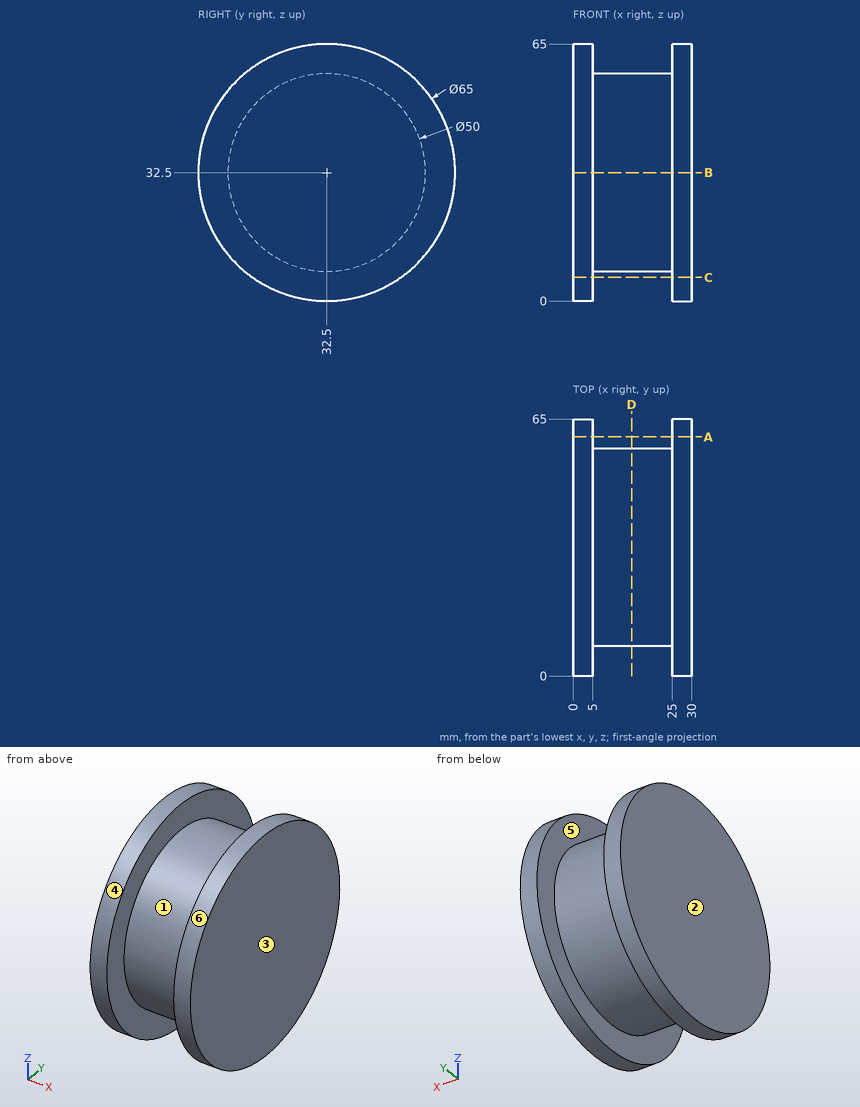
For this review, use the dimensioned drawing (mm, ordinates from the lowest corner) and the shaded views. A direction names the side the tool comes from. Round coordinates to 2 decimals unless told otherwise and drop trailing zeros. Loops run counter-clockwise (first coordinate to the right, second up) from the corner with the lowest first, then second, coordinate; pieces in that order, holes last. Notation, with made-up numbers: M -28.75,-13 L 17.25,-13 A24 cw 17.25,20 Z; hole C 88,8.5 d5. An arc over 180 degrees is marked long. Answer as a JSON object with one key per item and string values.
(1) Take a section at C-C on z = 6. Give the boundary of the cut face in (x, y).
Resolved:
{"outline": "M 0,13.69 L 5,13.69 L 5,51.31 L 0,51.31 Z; M 25,13.69 L 30,13.69 L 30,51.31 L 25,51.31 Z"}
(2) Clearance check with flat-ended pins moving along their axes: P1, Ø1.5, axis at x = 18, z = 48.5, coming from the -Y side; P2, Ø12, axis at x = 16.5, z = 21.5, coming from the -Y side; P3, Ø1.5, axis at x = 22.5, y = 55.5, coming from the -Z side. State where each tip first meets the part, or that it passes through.
Resolved:
{"P1": "y = 12.69", "P2": "y = 8.01", "P3": "z = 21.1"}
(3) Tool access review of the marked faces 5 and 6: name each direction out of +Z, -Z, +X, -X, +Y, -Y from which nothing blocks a thin tool from reaching the whole face with its end or side.
Resolved:
{"face 5": "none", "face 6": "+X, -X"}
(4) Take a section at B-B on z = 32.5. Give the boundary of the cut face in (x, y), and give its area (3 significant figures).
Resolved:
{"outline": "M 0,0 L 5,0 L 5,7.5 L 25,7.5 L 25,0 L 30,0 L 30,65 L 25,65 L 25,57.5 L 5,57.5 L 5,65 L 0,65 Z", "area": "1,650 mm²"}
(5) Draft analysis for pull direction X (two halves, no side actions). For the marked faces 1, 2, 3 and 4, state which applies: released by +X, released by -X, zero draft, split by the parting line, or undercut.
Resolved:
{"face 1": "undercut", "face 2": "released by -X", "face 3": "released by +X", "face 4": "zero draft"}
(6) Take a section at A-A on y = 60.5. Give the boundary of the cut face in (x, z), and give its area (3 significant figures).
Resolved:
{"outline": "M 0,16 L 5,16 L 5,49 L 0,49 Z; M 25,16 L 30,16 L 30,49 L 25,49 Z", "area": "330 mm²"}
(7) To check wall thickness, follow line 1 along X through (y, z) = (35, 4); line 2 along Z through (x, y) = (8, 43); line 3 along Y through (x, z) = (16.5, 21). State the ranges of each line that lie inside material, in increasing order.
Resolved:
{"line 1": "0 to 5, 25 to 30", "line 2": "9.81 to 55.19", "line 3": "10.3 to 54.7"}
(8) Take a section at D-D on x = 14.75. Give the boundary of the cut face in (y, z).
Resolved:
{"outline": "C 32.5,32.5 d50"}
